The model under review builds one solid part; all positions refer to its coordinate system, in mm. A direction names the side the tool comes from. Round coordinates to 2 decimals unless told otherwise and drop trailing zeros. Write each loop counter-clockwise with the first axis right and the second up, starting at its lowest first coordinate (ties: lowest second). Pieces come first, ordered by that corner, then holes. Notation, with made-up numbers: (81, 69.25) -> (124, 69.25) arc R18 ccw to (124, 100.25) -> close; hole circle Ø4 at (57, 3.25). An arc over 180 degrees is marked (long way). Return JSON: item names as keys, results as strings. Group by question number.
1. Take a section at B-B, the plane y = 41. Write out the cut boundary in (x, z).
2. Take a section at C-C, the plane z = 22.5. Write out the cut boundary in (x, y).
3. Clearance check with flat-ended pins moving along their axes: P1, Ø4, axis at y = 18.5, z = 18.5, coming from the +X side; P2, Ø10, axis at x = 21, y = 14.5, coming from the +Z side; P3, Ø6.5, axis at x = -28.75, z = 22.5, coming from the +Y side. State where each tip first meets the part, or that it passes through.
4. Take a section at D-D, the plane x = -28.75. Write out the cut boundary in (y, z).
5. Tool access review of faces 4 (the flat face through (19, 12, 2.5)), 5 (the flat face through (4.5, 39, -19)), 6 (the flat face through (-3, 41, -23)): name each direction out of +Z, -Z, +X, -X, +Y, -Y from which nothing blocks a thin tool from reaching the whole face with its end or side.
6. Take a section at A-A, the plane x = 7. Write out the cut boundary in (y, z).
7. For line 1 along X through (y, z) = (1.9, -22.5); line 2 along X through (y, z) = (7.5, 5.5); line 3 along Z through (x, y) = (3.5, 41), list the stretches that pass through material, from the lowest coordinate up. Write a range as from..to.
8. Mouldability with a two-part tool opening along Y and no side actions: class faces 1 (the flat face through (-38.75, 2, 0)), 2 (the cylindrical face through (-1.77, 40.01, -20.91)), 3 (the flat face through (-21, 18, 0)) as pulls with the +Y half, pulls with the -Y half, needs draft (parallel to the pull), parting line crosses it, or undercut.
from build123d import *

# Parameters (mm, degrees)
SKETCH1_W                = 77.5
SKETCH1_H                = 65
BOSS_EXTRUDE1_DEPTH      = 5
F_5_0_5_DIAMETER_HOLE1_D = 5
SKETCH4_W                = 30
SKETCH4_H                = 30
BOSS_EXTRUDE2_DEPTH      = 40
CUT_EXTRUDE1_REACH       = 69.696
SKETCH5_W                = 20.5
SKETCH5_H                = 20.5
BOSS_EXTRUDE3_DEPTH      = 2.5
CIRPATTERN1_COUNT        = 2
CIRPATTERN1_ANGLE        = 90
CIRPATTERN2_COUNT        = 2
CIRPATTERN2_ANGLE        = 90
CUT_EXTRUDE4_REACH       = 78.045
SKETCH11_W               = 1
SKETCH11_H               = 40
SKETCH12_W               = 4
SKETCH12_H               = 8
BOSS_EXTRUDE5_DEPTH      = 8
FILLET3_R                = 8
FILLET3_OF_MIRROR2_R     = 8
CUT_EXTRUDE5_REACH       = 72.369
SKETCH13_R               = 2.15
SKETCH14_R               = 2.75
CUT_EXTRUDE6_DEPTH       = 1.5
CUT_EXTRUDE7_REACH       = 72.369
SKETCH15_R               = 1.5
FILLET1_R                = 5


with BuildPart() as part:
    # Sketch1 → Boss-Extrude1 (new body)
    with BuildSketch(Plane(origin=(0, 0, 0), x_dir=(1, 0, 0), z_dir=(0, 1, 0))):
        Rectangle(SKETCH1_W, SKETCH1_H)
    extrude(amount=BOSS_EXTRUDE1_DEPTH)

    # Ø5.0 (5) Diameter Hole1 (through all)
    with Locations(Plane(origin=(-28.75, 5, -22.5), x_dir=(0, 0, 1), z_dir=(0, 1, 0))):
        with Locations((0, 0), (0, 57.5), (45, 57.5), (45, 0)):
            Hole(F_5_0_5_DIAMETER_HOLE1_D / 2)

    # Sketch4 → Boss-Extrude2 (add)
    with BuildSketch(Plane(origin=(0, 5, 0), x_dir=(1, 0, 0), z_dir=(0, 1, 0))):
        Rectangle(SKETCH4_W, SKETCH4_H)
    extrude(amount=BOSS_EXTRUDE2_DEPTH)

    # Sketch5 → Cut-Extrude1 (cut, up to next)
    with BuildSketch(Plane(origin=(0, 45, 0), x_dir=(1, 0, 0), z_dir=(0, 1, 0)), mode=Mode.PRIVATE) as cut_extrude1_sk1:
        Rectangle(SKETCH5_W, SKETCH5_H)
    cut_extrude1_tool1 = extrude(cut_extrude1_sk1.sketch, amount=-CUT_EXTRUDE1_REACH, mode=Mode.PRIVATE) & part.part
    add(cut_extrude1_tool1.solids().sort_by_distance((0, 45, 0))[0], mode=Mode.SUBTRACT)

    # Sketch7 → Boss-Extrude3 (add, symmetric)
    with BuildSketch(Plane(origin=(0, 0, 0), x_dir=(0, 0, -1), z_dir=(1, 0, 0))):
        Polygon((-15, 30), (-27.5, 5), (-15, 5), align=None)
    boss_extrude3 = extrude(amount=BOSS_EXTRUDE3_DEPTH, both=True)

    # CirPattern1: Boss-Extrude3 ×2 about axis
    cirpattern1_axis = Axis((0, 0, 0), (0, 1, 0))
    for i in range(1, CIRPATTERN1_COUNT):
        add(boss_extrude3.rotate(cirpattern1_axis, i * CIRPATTERN1_ANGLE / (CIRPATTERN1_COUNT - 1)))

    # CirPattern2: Boss-Extrude3 ×2 about axis
    cirpattern2_axis = Axis((0, 0, 0), (0, -1, 0))
    for i in range(1, CIRPATTERN2_COUNT):
        add(boss_extrude3.rotate(cirpattern2_axis, i * CIRPATTERN2_ANGLE / (CIRPATTERN2_COUNT - 1)))

    # Sketch11 → Cut-Extrude4 (cut, up to next)
    with BuildSketch(Plane(origin=(0, 0, -15), x_dir=(-1, 0, 0), z_dir=(0, 0, -1)), mode=Mode.PRIVATE) as cut_extrude4_sk1:
        with Locations((0, 25)):
            Rectangle(SKETCH11_W, SKETCH11_H)
    cut_extrude4_tool1 = extrude(cut_extrude4_sk1.sketch, amount=-CUT_EXTRUDE4_REACH, mode=Mode.PRIVATE) & part.part
    add(cut_extrude4_tool1.solids().sort_by_distance((0, 25, -15))[0], mode=Mode.SUBTRACT)

    # Sketch12 → Boss-Extrude5 (add)
    with BuildSketch(Plane(origin=(0, 0, -15), x_dir=(-1, 0, 0), z_dir=(0, 0, -1))):
        with Locations((-2.5, 41)):
            Rectangle(SKETCH12_W, SKETCH12_H)
    boss_extrude5 = extrude(amount=BOSS_EXTRUDE5_DEPTH)

    # Fillet3
    fillet3_edges = [part.edges().sort_by_distance(p)[0] for p in [
        (2.5, 37, -15),
    ]]
    fillet(fillet3_edges, radius=FILLET3_R - 0.0001)  # a hair under: the kernel refuses the full size

    # Mirror2: Boss-Extrude5 across plane
    add(boss_extrude5.mirror(Plane(origin=(0, 0, 0), x_dir=(0, 0, 1), z_dir=(1, 0, 0))))

    # Fillet3 of Mirror2
    fillet3_of_mirror2_edges = [part.edges().sort_by_distance(p)[0] for p in [
        (-2.5, 37, -15),
    ]]
    fillet(fillet3_of_mirror2_edges, radius=FILLET3_OF_MIRROR2_R - 0.0001)  # a hair under: the kernel refuses the full size

    # Sketch13 → Cut-Extrude5 (cut, up to next)
    with BuildSketch(Plane.ZY.offset(4.5), mode=Mode.PRIVATE) as cut_extrude5_sk1:
        with Locations(Location((-19, 41, 0), (0, 0, 270))):
            Circle(SKETCH13_R)
    cut_extrude5_tool1 = extrude(cut_extrude5_sk1.sketch, amount=-CUT_EXTRUDE5_REACH, mode=Mode.PRIVATE) & part.part
    add(cut_extrude5_tool1.solids().sort_by_distance((-4.5, 41, -19))[0], mode=Mode.SUBTRACT)

    # Sketch14 → Cut-Extrude6 (cut)
    with BuildSketch(Plane.ZY.offset(4.5)):
        with Locations(Location((-19, 41, 0), (0, 0, 270))):
            Circle(SKETCH14_R)
    extrude(amount=-CUT_EXTRUDE6_DEPTH, mode=Mode.SUBTRACT)

    # Sketch15 → Cut-Extrude7 (cut, up to next)
    with BuildSketch(Plane(origin=(4.5, 0, 0), x_dir=(0, 0, -1), z_dir=(1, 0, 0)), mode=Mode.PRIVATE) as cut_extrude7_sk1:
        with Locations(Location((19, 41, 0), (0, 0, 90))):
            Circle(SKETCH15_R)
    cut_extrude7_tool1 = extrude(cut_extrude7_sk1.sketch, amount=-CUT_EXTRUDE7_REACH, mode=Mode.PRIVATE) & part.part
    add(cut_extrude7_tool1.solids().sort_by_distance((4.5, 41, -19))[0], mode=Mode.SUBTRACT)

    # Fillet1
    fillet1_edges = [part.edges().sort_by_distance(p)[0] for p in [
        (-38.75, 2.5, -32.5),
        (38.75, 2.5, -32.5),
        (38.75, 2.5, 32.5),
        (-38.75, 2.5, 32.5),
    ]]
    fillet(fillet1_edges, radius=FILLET1_R)


solid = part.part
Output:
{
 "1": {"outline": "(-15, -15) -> (-4.5, -15) -> (-4.5, -16.25) -> (-3, -16.25) -> (-3, -16.85) -> (-0.5, -16.85) -> (-0.5, -10.25) -> (-10.25, -10.25) -> (-10.25, 10.25) -> (10.25, 10.25) -> (10.25, -10.25) -> (0.5, -10.25) -> (0.5, -17.5) -> (4.5, -17.5) -> (4.5, -15) -> (15, -15) -> (15, 15) -> (-15, 15) -> close; (-4.5, -23) -> (-0.5, -23) -> (-0.5, -21.15) -> (-3, -21.15) -> (-3, -21.75) -> (-4.5, -21.75) -> close; (0.5, -23) -> (4.5, -23) -> (4.5, -20.5) -> (0.5, -20.5) -> close"},
 "2": {"outline": "(-38.75, 0) -> (-31.25, 0) -> (-31.25, 5) -> (-38.75, 5) -> close; (-26.25, 0) -> (26.25, 0) -> (26.25, 5) -> (2.5, 5) -> (2.5, 15) -> (-2.5, 15) -> (-2.5, 5) -> (-26.25, 5) -> close; (31.25, 0) -> (38.75, 0) -> (38.75, 5) -> (31.25, 5) -> close"},
 "3": {"P1": "stops at x = 2.5", "P2": "stops at z = 2.5", "P3": "stops at y = 5"},
 "4": {"outline": "(0, -32.5) -> (5, -32.5) -> (5, -25) -> (0, -25) -> close; (0, -20) -> (5, -20) -> (5, 20) -> (0, 20) -> close; (0, 25) -> (5, 25) -> (5, 32.5) -> (0, 32.5) -> close"},
 "5": {"face 4": "+Z, +X, +Y", "face 5": "-Z, +X, +Y", "face 6": "-Z, +X, -X, +Y"},
 "6": {"outline": "(0, -32.5) -> (5, -32.5) -> (5, -15) -> (45, -15) -> (45, -10.25) -> (0, -10.25) -> close; (0, 10.25) -> (45, 10.25) -> (45, 15) -> (5, 15) -> (5, 32.5) -> (0, 32.5) -> close"},
 "7": {"line 1": "x = -38.75..-31.25, -26.25..26.25, 31.25..38.75", "line 2": "x = -15..-10.25, 10.25..15", "line 3": "z = -23..-20.5, -17.5..-10.25, 10.25..15"},
 "8": {"face 1": "needs draft", "face 2": "undercut", "face 3": "pulls with the +Y half"}
}
